Can you work these out from the model? Positions are in its coordinate system, mm. Face numbers are marked on the shaded views. A direction names the side the tool comes from. Coordinates: 2 decimals unless noted, no trailing zeros. Loops run counter-clockwise (first coordinate to the right, second up) from the corner with the lowest first, then second, coordinate; pieces in that order, holes last.
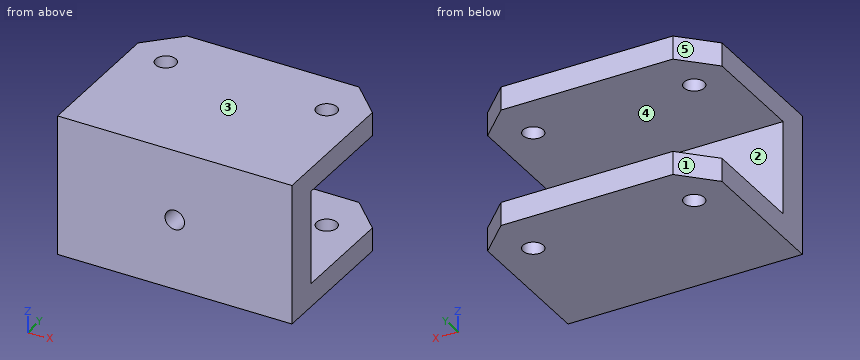
```python
from build123d import *

# Parameters (mm, degrees)
SKETCH_2_R          = 1.3
EXTRUDE_1_DEPTH     = 9
SKETCH_3_W          = 30
SKETCH_3_H          = 20.835575778
CUT_EXTRUDE_1_DEPTH = 6
CUT_EXTRUDE_2_REACH = 22.664
SKETCH_4_R          = 1.25


with BuildPart() as part:
    # 草图2 → 凸台-拉伸1 (new, symmetric)
    with BuildSketch(Plane.XY):
        Polygon((-11, 11), (11, 11), (15, 7), (15, -11), (-15, -11), (-15, 7), align=None)
        with Locations((-10.3, 5)):
            Circle(SKETCH_2_R, mode=Mode.SUBTRACT)
        with Locations(Location((10.3, 5, 0), (0, 0, 180))):
            Circle(SKETCH_2_R, mode=Mode.SUBTRACT)
    extrude(amount=EXTRUDE_1_DEPTH, both=True)

    # 草图3 → 切除-拉伸1 (cut, symmetric)
    with BuildSketch(Plane.XY):
        with Locations((0, 3.717787889)):
            Rectangle(SKETCH_3_W, SKETCH_3_H)
    extrude(amount=CUT_EXTRUDE_1_DEPTH, both=True, mode=Mode.SUBTRACT)

    # 草图4 → 切除-拉伸2 (cut, up to next)
    with BuildSketch(Plane(origin=(0, 0, 0), x_dir=(1, 0, 0), z_dir=(0, 1, 0)), mode=Mode.PRIVATE) as cut_extrude_2_sk1:
        with Locations(Location((0, 0, 0), (0, 0, 270))):
            Circle(SKETCH_4_R)
    cut_extrude_2_tool1 = extrude(cut_extrude_2_sk1.sketch, amount=-CUT_EXTRUDE_2_REACH, mode=Mode.PRIVATE) & part.part
    add(cut_extrude_2_tool1.solids().sort_by_distance((0, 0, 0))[0], mode=Mode.SUBTRACT)


solid = part.part
```
Item 1: We'd pull the mould along Z, two halves only. Please class the marked faces 3, 4 and 5: +Z half, -Z half, draft (parallel to the pull), parting line (faces both ways), or undercut.
Results are:
face 3: +Z half
face 4: undercut
face 5: draft
Item 2: I need wall thicknesses on line 1 along X through (y, z) = (5, 6.7); line 2 along Z through (x, y) = (-10.25, 9.25); line 3 along Y through (x, z) = (10.3, 7.65). Which ranges of each line are inside material? Lowest first, please.
Results are:
line 1: x = -15 to -11.6, -9 to 9, 11.6 to 15
line 2: z = -9 to -6, 6 to 9
line 3: y = -11 to 3.7, 6.3 to 11
Item 3: Suppose I cut it at D-D, the plane y = 5. Please give me the cut outline in (x, z), plus the area to 3 significant figures.
Results are:
outline: (-15, -9) - (-11.6, -9) - (-11.6, -6) - (-15, -6) - close; (-15, 6) - (-11.6, 6) - (-11.6, 9) - (-15, 9) - close; (-9, -9) - (9, -9) - (9, -6) - (-9, -6) - close; (-9, 6) - (9, 6) - (9, 9) - (-9, 9) - close; (11.6, -9) - (15, -9) - (15, -6) - (11.6, -6) - close; (11.6, 6) - (15, 6) - (15, 9) - (11.6, 9) - close
area: 149 mm2
Item 4: I'm going to push flat-ended pins straight in: P1, Ø10, axis at x = 2, z = 3.5, coming from the +Y side; P2, Ø2, axis at x = 7.5, z = -1, coming from the +Y side. Where does each tip first touch, or does it pass through?
Results are:
P1: stops at y = 11
P2: stops at y = -6.7
Item 5: Suppose I cut it at B-B, the plane z = 0. Please give me the cut outline in (x, y), plus the area to 3 significant figures.
Results are:
outline: (-15, -11) - (-1.25, -11) - (-1.25, -6.7) - (-15, -6.7) - close; (1.25, -11) - (15, -11) - (15, -6.7) - (1.25, -6.7) - close
area: 118 mm2
Item 6: Suppose I cut it at C-C, the plane x = 10.3. Please give me the cut outline in (y, z).
Results are:
outline: (-11, -9) - (3.7, -9) - (3.7, -6) - (-6.7, -6) - (-6.7, 6) - (3.7, 6) - (3.7, 9) - (-11, 9) - close; (6.3, -9) - (11, -9) - (11, -6) - (6.3, -6) - close; (6.3, 6) - (11, 6) - (11, 9) - (6.3, 9) - close
Item 7: On a 3-axis mill with a long thin cutter (end or side, diameter ignored), from which of +Z, -Z, +X, -X, +Y, -Y can I reach the whole of each face in a straight line? I mean the marked faces 1 and 2. Say none if no direction works.
Results are:
face 1: +Z, -Z, -X, +Y
face 2: +X, -X, +Y
Item 8: Suppose I cut it at A-A, the plane x = 0. Please give me the cut outline in (y, z).
Results are:
outline: (-11, -9) - (11, -9) - (11, -6) - (-6.7, -6) - (-6.7, -1.25) - (-11, -1.25) - close; (-11, 1.25) - (-6.7, 1.25) - (-6.7, 6) - (11, 6) - (11, 9) - (-11, 9) - close
